For this review, use the dimensioned drawing (mm, ordinates from the lowest corner) and the shaded views. Coordinates: 2 decimals unless noted, no trailing zeros. Order: outer loops, then holes, each group sorted by start corner. A loop starts at its lowest first (then second) coordinate and runs counter-clockwise, first axis right, second up. Notation, with made-up numbers: M 67,28.5 L 104,28.5 A28 cw 104,49.5 Z; hole C -40,27.25 d4. An arc over 180 degrees is marked long. Use one line per item in the form item = value. Start each with the question number.
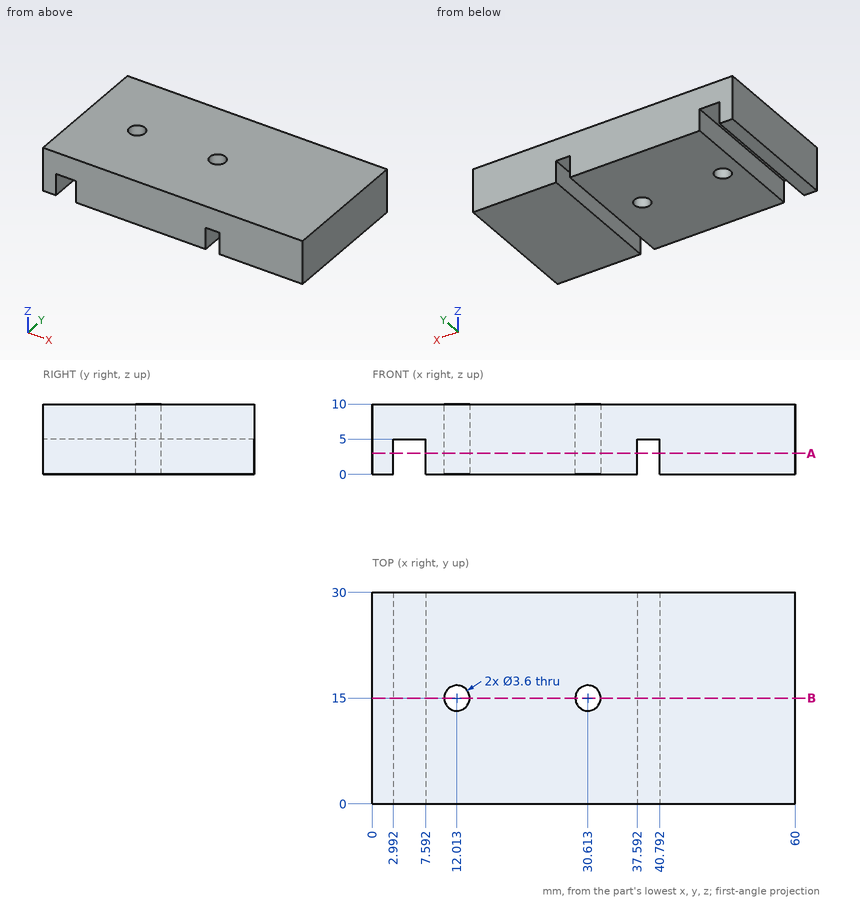
1. Consider section A-A, the plane z = 3. Write out the cut boundary in (x, y), plus the area to 3 significant figures.
2. For pin 1 Ø3 at (x, y) = (30.61, 15) entering from +Z; pin 2 Ø1.4 at (x, y) = (6, 7.5) entering from -Z, all flat-tipped, find the tip position at first contact; note any pin that passes through.
3. Consider section B-B, the plane y = 15. Write out the cut boundary in (x, z), plus the area to 3 significant figures.
4. To check wall thickness, follow line 1 (X direction, y = 19, z = 4.25); line 2 (Y direction, x = 12, z = 8.5); line 3 (Y direction, x = 12.5, z = 2). State the ranges of each line that lie inside material, in increasing order.
Answers follow:
q1.outline = M 0,0 L 2.99,0 L 2.99,30 L 0,30 Z; M 7.59,0 L 37.59,0 L 37.59,30 L 7.59,30 Z; M 40.79,0 L 60,0 L 60,30 L 40.79,30 Z; hole C 12.01,15 d3.6; hole C 30.61,15 d3.6
q1.area = 1,550 mm²
q2.pin_1 = through
q2.pin_2 = 5
q3.outline = M 0,0 L 2.99,0 L 2.99,5 L 7.59,5 L 7.59,0 L 10.21,0 L 10.21,10 L 0,10 Z; M 13.81,0 L 28.81,0 L 28.81,10 L 13.81,10 Z; M 32.41,0 L 37.59,0 L 37.59,5 L 40.79,5 L 40.79,0 L 60,0 L 60,10 L 32.41,10 Z
q3.area = 489 mm²
q4.line_1 = 0 to 2.99, 7.59 to 37.59, 40.79 to 60
q4.line_2 = 0 to 13.2, 16.8 to 30
q4.line_3 = 0 to 13.27, 16.73 to 30
